Geometry check sheet. Reference: the model listing, model coordinates, mm. Face numbers are marked on the shaded views. A direction names the side the tool comes from. Coordinates: 2 decimals unless noted, no trailing zeros. Order: outer loops, then holes, each group sorted by start corner. A loop starts at its lowest first (then second) coordinate and runs counter-clockwise, first axis right, second up. Notation, with made-up numbers: (-36.5, 5) - (-22.5, 5) arc R13 ccw to (-22.5, 15) - close; hole circle Ø1 at (42.5, 62). An arc over 180 degrees is marked (long way). Put each result on its own line as item: value.
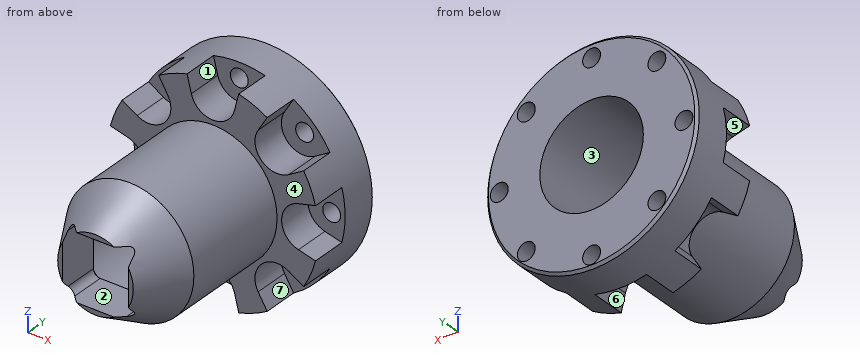
from build123d import *

# Parameters (mm, degrees)
F0_R      = 126
F1_DEPTH  = 275
F2_R      = 126
F2_R_2    = 76.45
F3_DEPTH  = 186.75
F4_R      = 10.625
F5_DEPTH  = 25
F6_DEPTH  = 169
F8_DEPTH  = 42
F9_SIZE   = 3
F10_R     = 61.65
F11_DEPTH = 218.05
F14_W     = 78.15
F14_H     = 78.15
F15_DEPTH = 60
F16_R     = 8
F17_R     = 8
F18_R     = 8
F19_R     = 8
F20_SIZE  = 8


with BuildPart() as f1:
    # F0 (on Front) → F1 (new body)
    with BuildSketch(Plane.XZ):
        Circle(F0_R)
    extrude(amount=F1_DEPTH)

    # F2 (on face) → F3 (cut)
    with BuildSketch(Plane.XZ.offset(275)):
        Circle(F2_R)
        Circle(F2_R_2, mode=Mode.SUBTRACT)
    extrude(amount=-F3_DEPTH, mode=Mode.SUBTRACT)

    # F4 (on face) → F5 (cut)
    with BuildSketch(Plane.XZ.offset(88.25)):
        with Locations((0, 108.3187091187)):
            Circle(F4_R)
        with Locations((-77.7817459305, 76.1004550493)):
            Circle(F4_R)
        with Locations((-110, -1.6812908813)):
            Circle(F4_R)
        with Locations((-77.7817459305, -79.4630368118)):
            Circle(F4_R)
        with Locations((0, -111.6812908813)):
            Circle(F4_R)
        with Locations((77.7817459305, -79.4630368118)):
            Circle(F4_R)
        with Locations((110, -1.6812908813)):
            Circle(F4_R)
        with Locations((77.7817459305, 76.1004550493)):
            Circle(F4_R)
    extrude(amount=-F5_DEPTH, mode=Mode.SUBTRACT)

    # F4 (on face) → F6 (cut)
    with BuildSketch(Plane.XZ.offset(88.25)):
        with Locations((0, 108.3187091187)):
            Circle(F4_R)
        with Locations((-77.7817459305, 76.1004550493)):
            Circle(F4_R)
        with Locations((-110, -1.6812908813)):
            Circle(F4_R)
        with Locations((-77.7817459305, -79.4630368118)):
            Circle(F4_R)
        with Locations((0, -111.6812908813)):
            Circle(F4_R)
        with Locations((77.7817459305, -79.4630368118)):
            Circle(F4_R)
        with Locations((110, -1.6812908813)):
            Circle(F4_R)
        with Locations((77.7817459305, 76.1004550493)):
            Circle(F4_R)
    extrude(amount=-F6_DEPTH, mode=Mode.SUBTRACT)

    # F7 (on face) → F8 (cut)
    with BuildSketch(Plane.XZ.offset(88.25)):
        with BuildLine():
            Line((-36.7983387241, 146.3692988564), (-25.7128367463, 101.9077788854))
            ThreePointArc((-25.7128367463, 101.9077788854), (0, 81.8187091187), (25.7128367463, 101.9077788854))
            Line((25.7128367463, 101.9077788854), (36.7983387241, 146.3692988564))
            Line((36.7983387241, 146.3692988564), (-36.7983387241, 146.3692988564))
        make_face()
        with BuildLine():
            Line((-53.8779602786, 90.2414027324), (-77.4783689307, 129.5190786271))
            Line((-77.4783689307, 129.5190786271), (-129.5190786271, 77.4783689307))
            Line((-129.5190786271, 77.4783689307), (-90.2414027324, 53.8779602786))
            ThreePointArc((-90.2414027324, 53.8779602786), (-57.8545640458, 57.8545640458), (-53.8779602786, 90.2414027324))
        make_face()
        with BuildLine():
            Line((-101.9077788854, 25.7128367463), (-146.3692988564, 36.7983387241))
            Line((-146.3692988564, 36.7983387241), (-146.3692988564, -36.7983387241))
            Line((-146.3692988564, -36.7983387241), (-101.9077788854, -25.7128367463))
            ThreePointArc((-101.9077788854, -25.7128367463), (-81.8187091187, 0), (-101.9077788854, 25.7128367463))
        make_face()
        with BuildLine():
            Line((-90.2414027324, -53.8779602786), (-129.5190786271, -77.4783689307))
            Line((-129.5190786271, -77.4783689307), (-77.4783689307, -129.5190786271))
            Line((-77.4783689307, -129.5190786271), (-53.8779602786, -90.2414027324))
            ThreePointArc((-53.8779602786, -90.2414027324), (-57.8545640458, -57.8545640458), (-90.2414027324, -53.8779602786))
        make_face()
        with BuildLine():
            Line((-25.7128367463, -101.9077788854), (-36.7983387241, -146.3692988564))
            Line((-36.7983387241, -146.3692988564), (36.7983387241, -146.3692988564))
            Line((36.7983387241, -146.3692988564), (25.7128367463, -101.9077788854))
            ThreePointArc((25.7128367463, -101.9077788854), (0, -81.8187091187), (-25.7128367463, -101.9077788854))
        make_face()
        with BuildLine():
            Line((53.8779602786, -90.2414027324), (77.4783689307, -129.5190786271))
            Line((77.4783689307, -129.5190786271), (129.5190786271, -77.4783689307))
            Line((129.5190786271, -77.4783689307), (90.2414027324, -53.8779602786))
            ThreePointArc((90.2414027324, -53.8779602786), (57.8545640458, -57.8545640458), (53.8779602786, -90.2414027324))
        make_face()
        with BuildLine():
            Line((101.9077788854, -25.7128367463), (146.3692988564, -36.7983387241))
            Line((146.3692988564, -36.7983387241), (146.3692988564, 36.7983387241))
            Line((146.3692988564, 36.7983387241), (101.9077788854, 25.7128367463))
            ThreePointArc((101.9077788854, 25.7128367463), (81.8187091187, 0), (101.9077788854, -25.7128367463))
        make_face()
        with BuildLine():
            Line((90.2414027324, 53.8779602786), (129.5190786271, 77.4783689307))
            Line((129.5190786271, 77.4783689307), (77.4783689307, 129.5190786271))
            Line((77.4783689307, 129.5190786271), (53.8779602786, 90.2414027324))
            ThreePointArc((53.8779602786, 90.2414027324), (57.8545640458, 57.8545640458), (90.2414027324, 53.8779602786))
        make_face()
    extrude(amount=-F8_DEPTH, mode=Mode.SUBTRACT)

    # F9
    f9_edges = [f1.edges().sort_by_distance(p)[0] for p in [
        (-126, 0, 0),
    ]]
    chamfer(f9_edges, length=F9_SIZE)

    # F10 (on face) → F11 (cut)
    with BuildSketch(Plane(origin=(0, 0, 0), x_dir=(-1, 0, 0), z_dir=(0, 1, 0))):
        Circle(F10_R)
    extrude(amount=-F11_DEPTH, mode=Mode.SUBTRACT)

    # F12 (on Right) → F13 (revolve, cut)
    with BuildSketch(Plane.YZ):
        Polygon((-287.4912917614, 86.0934704542), (-275, 45), (-210.72777727, 82.1075850946), align=None)
    revolve(axis=Axis((0, -206.6095604543, 0), (0, -1, 0)), mode=Mode.SUBTRACT)

    # F14 (on face) → F15 (cut)
    with BuildSketch(Plane.XZ.offset(275)):
        Rectangle(F14_W, F14_H)
    extrude(amount=-F15_DEPTH, mode=Mode.SUBTRACT)

    # F16
    f16_edges = [f1.edges().sort_by_distance(p)[0] for p in [
        (-39.075, -237.639237, -39.075),
    ]]
    fillet(f16_edges, radius=F16_R)

    # F17
    f17_edges = [f1.edges().sort_by_distance(p)[0] for p in [
        (39.075, -237.639237, 39.075),
    ]]
    fillet(f17_edges, radius=F17_R)

    # F18
    f18_edges = [f1.edges().sort_by_distance(p)[0] for p in [
        (-39.075, -237.639237, 39.075),
    ]]
    fillet(f18_edges, radius=F18_R)

    # F19
    f19_edges = [f1.edges().sort_by_distance(p)[0] for p in [
        (39.075, -237.639237, -39.075),
    ]]
    fillet(f19_edges, radius=F19_R)

    # F20
    f20_edges = [f1.edges().sort_by_distance(p)[0] for p in [
        (-39.075, -218.05, 0),
        (-36.731854, -218.05, 36.731854),
        (0, -218.05, 39.075),
        (36.731854, -218.05, 36.731854),
        (39.075, -218.05, 0),
        (0, -218.05, -39.075),
        (-36.731854, -218.05, -36.731854),
        (36.731854, -218.05, -36.731854),
    ]]
    chamfer(f20_edges, length=F20_SIZE)


solid = f1.part
Q1. Access from +Z, -Z, +X, -X, +Y, -Y to the whole of each face (thin tool, end or side, straight path). Record for the marked faces 1, 2, 3 and 4.
Answer block:
face 1: +Z, -Y
face 2: +Y, -Y
face 3: +Y
face 4: -Y
Q2. Section check B-B on x = 0. State how many separate pieces and enclosed holes the cut face has, then the cut area to 3 significant figures.
Answer block:
separate pieces: 4
enclosed holes: 0
area: 12,000 mm^2
Q3. Section check D-D on y = -127.5. Record the boundary of the cut face in (x, z).
Answer block:
outline: circle Ø152.9 at (0, 0); hole circle Ø123.3 at (0, 0)
Q4. Depth check by flat-ended pin: pin 1 Ø8 at (x, z) = (-10.5, 37) entering from +Y (3 decimals); pin 2 Ø14.5 at (x, y) = (-4.5, -258.5) entering from -Z; pin 3 Ø14.5 at (y, z) = (-249.5, -11) entering from -X; pin 4 Ø19 at (x, z) = (77.78, 76.1) entering from +Y. Enter the tip coordinate at first touch or a pass-through.
Answer block:
pin 1: stops at y = -224.125
pin 2: stops at z = -58.57
pin 3: stops at x = -63.11
pin 4: passes through
Q5. Draft check along X on the marked faces 5, 6 and 7. Enter one of: pulls with the +X half, pulls with the -X half, needs draft (parallel to the pull), parting line crosses it, or undercut.
Answer block:
face 5: pulls with the -X half
face 6: undercut
face 7: pulls with the +X half
Q6. Section check C-C on y = -251. Record the boundary of the cut face in (x, z) (3 decimals), then the cut area to 3 significant figures.
Answer block:
outline: circle Ø117.713 at (0, 0); hole (-39.075, -31.075) arc R8 ccw to (-31.075, -39.075) - (31.075, -39.075) arc R8 ccw to (39.075, -31.075) - (39.075, 31.075) arc R8 ccw to (31.075, 39.075) - (-31.075, 39.075) arc R8 ccw to (-39.075, 31.075) - close
area: 4,830 mm^2
Q7. Thickness scan on L1, parallel to Z at x = 0, y = -24; L2, parallel to Z at x = 0, y = -117.5; L3, parallel to Z at x = -35.5, y = -220.5. Record the ranges inside material, lowest first. Write a range as [from, to].
Answer block:
L1: z = [-126, -122.31], [-101.06, -61.65], [61.65, 97.69], [118.94, 126]
L2: z = [-76.45, -61.65], [61.65, 76.45]
L3: z = [-67.71, -43.88], [43.88, 67.71]
